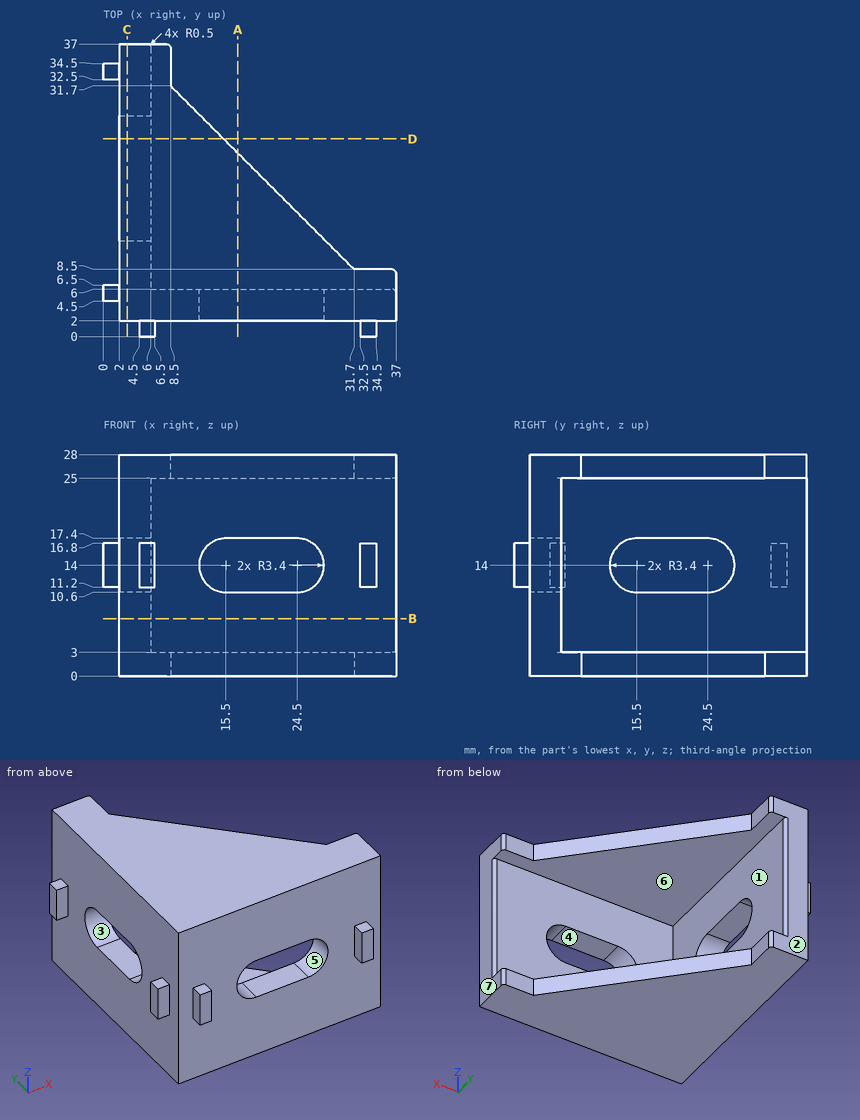
For this review, use the dimensioned drawing (mm, ordinates from the lowest corner) and the shaded views. A direction names the side the tool comes from. Round coordinates to 2 decimals unless told otherwise and drop trailing zeros. Order: outer loops, then holes, each group sorted by start corner. A loop starts at its lowest first (then second) coordinate and runs counter-clockwise, first axis right, second up. Notation, with made-up numbers: (67, -19) -> (98, -19) arc R26 ccw to (98, 8) -> close; hole circle Ø2 at (13, 1). An arc over 180 degrees is marked (long way). Write item = value, one per line. Start each with the question number.
Item 1: Clearance check with flat-ended pins moving along their axes: pin 1 Ø4 at (x, z) = (22, 20.5) entering from +Y; pin 2 Ø2 at (x, y) = (20, 4.5) entering from -Z; pin 3 Ø1.6 at (y, z) = (1, 12.5) entering from -X; pin 4 Ø1 at (x, y) = (33.5, 0.5) entering from -Z. State where each tip first meets the part, or that it passes through.
Item 2: For line 1 along Z through (x, y) = (11.5, 13); line 2 along X through (y, z) = (2.5, 8.25); line 3 along Y through (x, z) = (35.5, 8.5), list the stretches that pass through material, from the lowest coordinate up.
Item 3: Consider section B-B on z = 7.25. Write out the cut boundary in (x, y), plus the area to 3 significant figures.
Item 4: Consider section A-A on x = 17. Write out the cut boundary in (y, z).
Item 5: For the marked faces 1, 2, 3 and 4, list the 3-axis set-ups (+Z, -Z, +X, -X, +Y, -Y) from which the entire face can be reached by the end or side of a thin tool; tool diameter is ignored.
Item 6: Consider section C-C on x = 3. Write out the cut boundary in (y, z).
Item 7: Consider section D-D on y = 25. Write out the cut boundary in (x, z), plus the area to 3 significant figures.
Item 8: Mouldability with a two-part tool opening along X and no side actions: class the marked faces 5, 6 and 7 as released by +X, released by -X, zero draft, split by the parting line, or undercut.
Conclusion:
q1.pin_1 = 6
q1.pin_2 = 0
q1.pin_3 = 4.5
q1.pin_4 = 11.2
q2.line_1 = 0 to 3, 25 to 28
q2.line_2 = 2 to 37
q2.line_3 = 2 to 6
q3.outline = (2, 2) -> (37, 2) -> (37, 5.5) arc R0.5 ccw to (36.5, 6) -> (6, 6) -> (6, 36.5) arc R0.5 ccw to (5.5, 37) -> (2, 37) -> close
q3.area = 264 mm2
q4.outline = (2, 0) -> (23.2, 0) -> (23.2, 3) -> (6, 3) -> (6, 10.6) -> (2, 10.6) -> close; (2, 17.4) -> (6, 17.4) -> (6, 25) -> (23.2, 25) -> (23.2, 28) -> (2, 28) -> close
q5.face_1 = +X, +Y
q5.face_2 = +Z, -Z, +X, -X, +Y
q5.face_3 = +X, -X
q5.face_4 = +Y, -Y
q6.outline = (2, 0) -> (37, 0) -> (37, 28) -> (2, 28) -> close; hole (15.5, 10.6) -> (24.5, 10.6) arc R3.4 ccw to (24.5, 17.4) -> (15.5, 17.4) arc R3.4 ccw to start
q7.outline = (2, 0) -> (15.2, 0) -> (15.2, 3) -> (6, 3) -> (6, 10.64) -> (2, 10.64) -> close; (2, 17.36) -> (6, 17.36) -> (6, 25) -> (15.2, 25) -> (15.2, 28) -> (2, 28) -> close
q7.area = 140 mm2
q8.face_5 = undercut
q8.face_6 = zero draft
q8.face_7 = released by +X
